from build123d import *

# Parameters (mm, degrees)
F0_W     = 133
F0_H     = 50
F1_DEPTH = 2
F2_W     = 15
F2_H     = 7
F3_DEPTH = 4
F4_R     = 1.99999


# Not quite as in the source:
# - a fillet or chamfer is up to 0.001 mm smaller than in the source, because OpenCascade refuses the exact size


with BuildPart() as f1:
    # F0 (on Top) → F1 (new body)
    with BuildSketch(Plane.XY):
        Rectangle(F0_W, F0_H)
    extrude(amount=F1_DEPTH)

    # F2 (on face) → F3 (join)
    with BuildSketch(Plane(origin=(0, 0, 0), x_dir=(1, 0, 0), z_dir=(0, 0, -1))):
        with Locations((57, -19.5)):
            Rectangle(F2_W, F2_H)
    extrude(amount=F3_DEPTH)

    # F4 (radius 2 in the source; OpenCascade refuses exactly that, so slightly less here)
    f4_edges = [f1.edges().sort_by_distance(p)[0] for p in [
        (66.5, 25, 1),
        (66.5, -25, 1),
        (-66.5, 25, 1),
        (-66.5, -25, 1),
        (66.5, 0, 2),
        (0, 25, 2),
        (-66.5, 0, 2),
        (0, -25, 2),
    ]]
    fillet(f4_edges, radius=F4_R)


solid = f1.part
Can you work these out from the model? Positions are in its coordinate system, mm. A direction names the side the tool comes from. Coordinates: 2 decimals unless noted, no trailing zeros. Order: outer loops, then holes, each group sorted by start corner. A loop starts at its lowest first (then second) coordinate and runs counter-clockwise, first axis right, second up. Notation, with made-up numbers: (-12.75, 3.5) - (39.25, 3.5) arc R14 cw to (39.25, 22.5) - close; hole circle Ø6 at (-37, 49.25). An arc over 180 degrees is marked (long way). Answer as a JSON object with one key per item and string values. Group by question number.
Q1. Imagine slicing it at A-A (z = 1.1). Please give me the cut outline in (x, y).
Q2. Will these pins go through, and if not, where does the flat tip stop? P1, Ø1, axis at y = -20, z = 1, coming from the -X side; P2, Ø3, axis at x = -22, z = -2.5, coming from the +Y side; P3, Ø3, axis at y = 19, z = -2.5, coming from the +X side; P4, Ø5, axis at x = -2.5, y = -16, coming from the -Z side.
Q3. On a 3-axis mill with a long thin cutter (end or side, diameter ignored), from which of +Z, -Z, +X, -X, +Y, -Y can I reach the whole of each face in a straight line? I mean faces 1 (the face through (64.5, 20, -2)), 2 (the face through (49.5, 20, -2)), 3 (the face through (57, 19, -4)), 4 (the face through (57, 16, -2)), 5 (the face through (57, 23, -2)). Say none if no direction works.
Q4. I need wall thicknesses on line 1 (Z direction, x = 38.5, y = 7.5); line 2 (X direction, y = 18, z = 0.25); line 3 (X direction, y = 22, z = -0.4). Which ranges of each line are inside material? Lowest first, please. Write a range as from..to.
Determined:
{
 "1": {"outline": "(-66.17, -23) arc R1.67 ccw to (-64.5, -24.67) - (64.5, -24.67) arc R1.67 ccw to (66.17, -23) - (66.17, 23) arc R1.67 ccw to (64.5, 24.67) - (-64.5, 24.67) arc R1.67 ccw to (-66.17, 23) - close"},
 "2": {"P1": "stops at x = -66.44", "P2": "passes through", "P3": "stops at x = 64.5", "P4": "stops at z = 0"},
 "3": {"face 1": "-Z, +X, +Y, -Y", "face 2": "-Z, -X, +Y, -Y", "face 3": "-Z, +X, -X, +Y, -Y", "face 4": "-Z, +X, -X, -Y", "face 5": "-Z, +X, -X, +Y"},
 "4": {"line 1": "z = 0..2", "line 2": "x = -66.48..66.48", "line 3": "x = 49.5..64.5"}
}
